Verification items for the finished model (mm, model axes). A direction names the side the tool comes from. Round coordinates to 2 decimals unless told otherwise and drop trailing zeros. Write each loop counter-clockwise with the first axis right and the second up, starting at its lowest first coordinate (ties: lowest second). Pieces come first, ordered by that corner, then holes. Notation, with made-up numbers: (33, 46) -> (58, 46) arc R16 cw to (58, 55) -> close; hole circle Ø7 at (37, 30). An arc over 180 degrees is marked (long way). Use CSV: the item, a comma, the result in double quotes.
Autodesk Inventor part; units mm, degrees
ref_plane "YZ Plane" through (0, 0, 0) normal (1, 0, 0) x (0, 1, 0)
ref_plane "XZ Plane" through (0, 0, 0) normal (0, 1, 0) x (-1, 0, 0)
ref_plane "XY Plane" through (0, 0, 0) normal (0, 0, 1) x (1, 0, 0)
sketch "Sketch4" plane through (0, 0, 0) normal (0, 1, 0) x (-1, 0, 0)
  line L0 (63, -132.5) -> (-63, -132.5)
  line L1 (-63, -132.5) -> (-63, 132.5)
  line L2 (-63, 132.5) -> (63, 132.5)
  line L3 (63, 132.5) -> (63, -132.5)
  line L4 (63, -132.5) -> (-63, 132.5) construction
  point P0 (0, 0)
  point P1 (0, 0)
  dimension "d24" = 126
  dimension "d25" = 265
extrude "Plate4" add sketch "Sketch4" along normal mid plane 2
sketch "Sketch7" plane through (0, -1, 0) normal (0, -1, 0) x (1, 0, 0)
  circle A0 centre (46, -117.5) radius 5
  line L0 (63, 132.5) -> (63, -132.5)
  line L1 (63, -132.5) -> (-63, -132.5)
  line L2 (0, -74.3103) -> (0, 74.3103) construction
  line L3 (114.9724, 0) -> (-114.9724, 0) construction
  circle A1 centre (-46, -117.5) radius 5
  circle A2 centre (46, -32.5) radius 5
  circle A3 centre (-46, -32.5) radius 5
  point P0 (0, 0)
  point P1 (0, 0)
  dimension "d41" = 10
  dimension "d42" = 17
  dimension "d43" = 15
  dimension "d46" = 85
extrude "Extrusion2" cut sketch "Sketch7" against normal up to surface (2 mm away)
sketch "Sketch8" plane through (61, 1, 132.5) normal (1, 0, 0) x (0, 1, 0)
  line L0 (0, -265) -> (0, 0)
  line L1 (0, 0) -> (-25, 0)
  line L2 (-25, 0) -> (-25, -265)
  line L3 (-25, -265) -> (0, -265)
edge flange "Flange4" height 25 angle 90 thickness 2 bend radius 2 thickness toward (1, 0, 0) relief tear relief width 2 relief depth 1 corner gap 2 corner form 0 edges at (63, -1, 0) (-63, -1, 0) wall of the first edge with corners at (61, 1, -132.5) (61, 1, 132.5) (61, -24, 132.5) (61, -24, -132.5)
bend "Bend4"
corner "Corner4"
equation "\"d26\" = Thickness"
equation "\"d47\" = BendReliefWidth"
equation "\"d48\" = BendReliefDepth"
equation "\"d49\" = MinimumRemnant"
equation "\"d50\" = TransitionRadius"
equation "\"d53\" = BendRadius"
equation "\"d54\" = CornerReliefSize"
equation "\"d55\" = GapSize"
equation "\"d56\" = JacobiRadiusSize"
equation "\"BendRadius\" = Thickness"
equation "\"BendReliefWidth\" = Thickness"
equation "\"BendReliefDepth\" = 0.5 * Thickness"
equation "\"CornerReliefSize\" = 4 * Thickness"
equation "\"MinimumRemnant\" = 2 * Thickness"
equation "\"TransitionRadius\" = BendRadius"
equation "\"JacobiRadiusSize\" = BendRadius"
equation "\"GapSize\" = Thickness"
properties part number "Крепление"
Q1. Section check B-B (y = -17.25). Record the cut outline in (x, z), plus the area to 3 significant figures.
Filled in:
outline,"(-63, -132.5) -> (-61, -132.5) -> (-61, 132.5) -> (-63, 132.5) -> close; (61, -132.5) -> (63, -132.5) -> (63, 132.5) -> (61, 132.5) -> close"
area,"1,060 mm²"
Q2. Section check A-A (x = 46). Record the cut outline in (y, z).
Filled in:
outline,"(-1, -132.5) -> (1, -132.5) -> (1, -122.5) -> (-1, -122.5) -> close; (-1, -112.5) -> (1, -112.5) -> (1, -37.5) -> (-1, -37.5) -> close; (-1, -27.5) -> (1, -27.5) -> (1, 132.5) -> (-1, 132.5) -> close"
Q3. Section check C-C (z = -32.5). Record the cut outline in (x, y), plus the area to 3 significant figures.
Filled in:
outline,"(-63, -24) -> (-61, -24) -> (-61, -3) arc R2 cw to (-59, -1) -> (-51, -1) -> (-51, 1) -> (-59, 1) arc R4 ccw to (-63, -3) -> close; (-41, -1) -> (41, -1) -> (41, 1) -> (-41, 1) -> close; (51, -1) -> (59, -1) arc R2 cw to (61, -3) -> (61, -24) -> (63, -24) -> (63, -3) arc R4 ccw to (59, 1) -> (51, 1) -> close"
area,"299 mm²"
Q4. Access from +Z, -Z, +X, -X, +Y, -Y to the whole of each face (thin tool, end or side, straight path). Record for faces 1 (the flat face through (1, -1, 2)), 2 (the flat face through (-63, -14, -2)).
Filled in:
face 1,"+Z, -Z, -Y"
face 2,"+Z, -Z, -X, +Y, -Y"
Q5. Section check D-D (z = 111). Record the cut outline in (x, y).
Filled in:
outline,"(-63, -24) -> (-61, -24) -> (-61, -3) arc R2 cw to (-59, -1) -> (59, -1) arc R2 cw to (61, -3) -> (61, -24) -> (63, -24) -> (63, -3) arc R4 ccw to (59, 1) -> (-59, 1) arc R4 ccw to (-63, -3) -> close"
Q6. Go/stop test with a flat-tipped pin: P1, Ø4, axis at x = -49, z = -13, coming from the -Y side. Record where the tip stops, or that it passes through.
Filled in:
P1,"y = -1"
Q7. Mould release check, pull along Z, two halves, no side actions. Record for faces 3 (the cylindrical face through (-50, 0, -35.5)), 4 (the flat face through (0, 0, 132.5)), 5 (the flat face through (61, -13, 2)), 6 (the flat face through (0, 0, -132.5)): released by +Z, released by -Z, zero draft, split by the parting line, or undercut.
Filled in:
face 3,"undercut"
face 4,"released by +Z"
face 5,"zero draft"
face 6,"released by -Z"
Q8. Material ranges on L1, parallel to Z at x = -46, y = -0.6; L2, parallel to X at y = -15, z = 82; L3, parallel to Y at x = 32.5, z = -99, recorded low to high.
Filled in:
L1,"-132.5 to -122.5, -112.5 to -37.5, -27.5 to 132.5"
L2,"-63 to -61, 61 to 63"
L3,"-1 to 1"
